```python
from build123d import *

# Parameters (mm, degrees)
SKETCH1_W           = 60
SKETCH1_H           = 40
BOSS_EXTRUDE1_DEPTH = 3
SKETCH2_W           = 40
SKETCH2_H           = 20
CUT_EXTRUDE1_DEPTH  = 3
SKETCH3_R           = 2
CUT_EXTRUDE2_DEPTH  = 3
FILLET2_R           = 1
SKETCH4_W           = 20
SKETCH4_H           = 6
CUT_EXTRUDE3_DEPTH  = 3


with BuildPart() as part:
    # Sketch1 → Boss-Extrude1 (new body)
    with BuildSketch(Plane(origin=(0, 0, 0), x_dir=(1, 0, 0), z_dir=(0, 1, 0))):
        Rectangle(SKETCH1_W, SKETCH1_H)
    extrude(amount=BOSS_EXTRUDE1_DEPTH)

    # Sketch2 → Cut-Extrude1 (cut)
    with BuildSketch(Plane(origin=(0, 3, 0), x_dir=(1, 0, 0), z_dir=(0, 1, 0))):
        Rectangle(SKETCH2_W, SKETCH2_H)
    extrude(amount=-CUT_EXTRUDE1_DEPTH, mode=Mode.SUBTRACT)

    # Sketch3 → Cut-Extrude2 (cut)
    with BuildSketch(Plane(origin=(0, 3, 0), x_dir=(1, 0, 0), z_dir=(0, 1, 0))):
        with Locations(Location((25, 5, 0), (0, 0, 270))):
            Circle(SKETCH3_R)
        with Locations(Location((25, -5, 0), (0, 0, 90))):
            Circle(SKETCH3_R)
        with Locations(Location((-25, -5, 0), (0, 0, 270))):
            Circle(SKETCH3_R)
        with Locations(Location((-25, 5, 0), (0, 0, 90))):
            Circle(SKETCH3_R)
    extrude(amount=-CUT_EXTRUDE2_DEPTH, mode=Mode.SUBTRACT)

    # Fillet2
    fillet2_edges = [part.edges().sort_by_distance(p)[0] for p in [
        (-30, 1.5, -20),
        (30, 1.5, -20),
    ]]
    fillet(fillet2_edges, radius=FILLET2_R)

    # Sketch4 → Cut-Extrude3 (cut)
    with BuildSketch(Plane(origin=(0, 3, 0), x_dir=(1, 0, 0), z_dir=(0, 1, 0))):
        with Locations((0, -20)):
            Rectangle(SKETCH4_W, SKETCH4_H)
    extrude(amount=-CUT_EXTRUDE3_DEPTH, mode=Mode.SUBTRACT)


solid = part.part
```
For this review, take the finished solid that the model builds, in its own axes (mm). A direction names the side the tool comes from. Give positions to 0.01 mm unless a question says otherwise; leave off trailing zeros. Loops run counter-clockwise (first coordinate to the right, second up) from the corner with the lowest first, then second, coordinate; pieces in that order, holes last. Notation, with made-up numbers: M 43,25.25 L 71,25.25 A6 ccw 71,33.25 Z; hole C 16,37 d7. An arc over 180 degrees is marked long. One line per item, written item: value. Start each with the question number.
Q1. Add section C-C (y = 2.4). Give the boundary of the cut face in (x, z).
Q2. Clearance check with a flat-ended pin moving along its axis: pin 1 Ø0.9 at (x, y) = (-2.5, 2) entering from +Z. State where the tip first meets the part, or that it passes through.
Q3. Machinability: for faces 1 (the face through (-20, 2, 0)), 2 (the face through (0, 2, 17)), 3 (the face through (-7, 0, -14)), which of the approach directions +Z, -Z, +X, -X, +Y, -Y give a long, thin tool a straight path to every point of the face, cutting with its end or side? Answer none if there is none.
Q4. Draft analysis for pull direction X (two halves, no side actions). For faces 4 (the face through (0, 2, -10)), 5 (the face through (-20, 1, 20)), 6 (the face through (20, 2, 0)), 7 (the face through (30, 1, 1)), state which applies: released by +X, released by -X, zero draft, split by the parting line, or undercut.
Q5. Add section D-D (x = 25). Give the boundary of the cut face in (y, z), and give its area (3 significant figures).
Q6. Add section B-B (z = 0). Give the boundary of the cut face in (x, y), and give its area (3 significant figures).
Q7. Add section A-A (x = 12). Give the boundary of the cut face in (y, z).
Q8. For L1, parallel to X at y = 1.85, z = 5; L2, parallel to X at y = 2.55, z = -9.5; L3, parallel to Z at x = -5.5, y = 0.8, list the stretches that pass through material, from the lowest coordinate up.
Reply:
1. outline: M -30,-19 A1 ccw -29,-20 L 29,-20 A1 ccw 30,-19 L 30,20 L 10,20 L 10,17 L -10,17 L -10,20 L -30,20 Z; hole C -25,-5 d4; hole C -25,5 d4; hole M -20,-10 L 20,-10 L 20,10 L -20,10 Z; hole C 25,-5 d4; hole C 25,5 d4
2. pin 1: z = 17
3. face 1: +Y, -Y
3. face 2: +Z, +Y, -Y
3. face 3: +Z, -Z, +X, -X, -Y
4. face 4: undercut
4. face 5: zero draft
4. face 6: undercut
4. face 7: released by +X
5. outline: M 0,-20 L 3,-20 L 3,-7 L 0,-7 Z; M 0,-3 L 3,-3 L 3,3 L 0,3 Z; M 0,7 L 3,7 L 3,20 L 0,20 Z
5. area: 96.0 mm²
6. outline: M -30,0 L -20,0 L -20,3 L -30,3 Z; M 20,0 L 30,0 L 30,3 L 20,3 Z
6. area: 60.0 mm²
7. outline: M 0,-20 L 3,-20 L 3,-10 L 0,-10 Z; M 0,10 L 3,10 L 3,20 L 0,20 Z
8. L1: -30 to -27, -23 to -20, 20 to 23, 27 to 30
8. L2: -30 to -20, 20 to 30
8. L3: -20 to -10, 10 to 17
